Can you work these out from the model? Positions are in its coordinate system, mm. Round coordinates to 2 decimals unless told otherwise and drop trailing zeros. Write item = value, one per line.
from build123d import *

# Parameters (mm, degrees)
SKETCH_1_R          = 1.6
EXTRUDE_1_DEPTH     = 4
SKETCH_2_R          = 1.6
CUT_EXTRUDE_1_DEPTH = 3


with BuildPart() as part:
    # 草图1 → 凸台-拉伸1 (new body)
    with BuildSketch(Plane(origin=(0, 0, 0), x_dir=(1, 0, 0), z_dir=(0, 1, 0))):
        with BuildLine():
            Line((-176.25, 50), (176.25, 50))
            ThreePointArc((176.25, 50), (183.321067812, 47.071067812), (186.25, 40))
            Line((186.25, 40), (186.25, -40))
            ThreePointArc((186.25, -40), (183.321067812, -47.071067812), (176.25, -50))
            Line((176.25, -50), (-176.25, -50))
            ThreePointArc((-176.25, -50), (-183.321067812, -47.071067812), (-186.25, -40))
            Line((-186.25, -40), (-186.25, 40))
            ThreePointArc((-186.25, 40), (-183.321067812, 47.071067812), (-176.25, 50))
        make_face()
        with Locations(Location((181.25, -38, 0), (0, 0, 270))):
            Circle(SKETCH_1_R, mode=Mode.SUBTRACT)
        with Locations(Location((181.25, 37, 0), (0, 0, 270))):
            Circle(SKETCH_1_R, mode=Mode.SUBTRACT)
        with Locations(Location((-181.25, -38, 0), (0, 0, 90))):
            Circle(SKETCH_1_R, mode=Mode.SUBTRACT)
        with Locations(Location((-181.25, 37, 0), (0, 0, 90))):
            Circle(SKETCH_1_R, mode=Mode.SUBTRACT)
    extrude(amount=EXTRUDE_1_DEPTH)

    # 草图2 → 切除-拉伸1 (cut)
    with BuildSketch(Plane(origin=(0, 4, 0), x_dir=(1, 0, 0), z_dir=(0, 1, 0))):
        with Locations(Location((-15, -30, 0), (0, 0, 270))):
            Circle(SKETCH_2_R)
        with Locations(Location((15, -30, 0), (0, 0, 270))):
            Circle(SKETCH_2_R)
        with Locations(Location((15, -40, 0), (0, 0, 270))):
            Circle(SKETCH_2_R)
        with Locations(Location((-15, -40, 0), (0, 0, 270))):
            Circle(SKETCH_2_R)
        with Locations(Location((-5, -30, 0), (0, 0, 270))):
            Circle(SKETCH_2_R)
        with Locations(Location((5, -30, 0), (0, 0, 270))):
            Circle(SKETCH_2_R)
        with Locations(Location((-5, -40, 0), (0, 0, 270))):
            Circle(SKETCH_2_R)
        with Locations(Location((5, -40, 0), (0, 0, 270))):
            Circle(SKETCH_2_R)
    extrude(amount=-CUT_EXTRUDE_1_DEPTH, mode=Mode.SUBTRACT)


solid = part.part
(1) Will this pin go through, and if not, where does the flat tip stop? P1, Ø3, axis at x = 15, z = 40, coming from the +Y side.
Computed:
P1 = 1
(2) Thinking about a two-plate mould opening in Z: for faces 1 (the face through (183.4, 1.97, 46.99)), 2 (the face through (3, 4, -1)), 3 (the face through (183.24, 1.97, -47.15)), which applies, +Z half, -Z half, draft (parallel to the pull), parting line (faces both ways), or undercut?
Computed:
face_1 = +Z half
face_2 = draft
face_3 = -Z half
(3) If I drill on line 1 (X direction, y = 2.15, z = 40); line 2 (X direction, y = 2.1, z = -37); line 3 (Z direction, x = 15.5, y = 1.05), over which ranges is the centre line in solid material (lowest first)? Write a range as from..to.
Computed:
line_1 = -186.25..-16.6, -13.4..-6.6, -3.4..3.4, 6.6..13.4, 16.6..186.25
line_2 = -186.25..-182.85, -179.65..179.65, 182.85..186.25
line_3 = -50..28.48, 31.52..38.48, 41.52..50
